Design review of the part shown in the three views and the two pictorial views. Dimensions are in mm from the part's minimum x, y and z. Coordinates: 2 decimals unless noted, no trailing zeros. Loops run counter-clockwise (first coordinate to the right, second up) from the corner with the lowest first, then second, coordinate; pieces in that order, holes last.
Q1. Wall thickness on probe 1 along X at (y, z) = (14.75, 1.5); probe 2 along Y at (x, z) = (16, 3.75); probe 3 along X at (y, z) = (12.5, 9.5): over which ranges is each line inside the solid? List them lowest first.
Q2. For P1, Ø3, axis at x = 465, y = 22.5, coming from the -Z side, flat-tipped, find the tip position at first contact; note if it passes through.
Q3. Add section C-C on x = 524. Give the boundary of the cut face in (y, z), and give its area (3 significant figures).
Q4. Add section A-A on y = 15. Give the boundary of the cut face in (x, z), and give its area (3 significant figures).
Q5. Add section B-B on z = 7.25. Give the boundary of the cut face in (x, y), and give its area (3 significant figures).
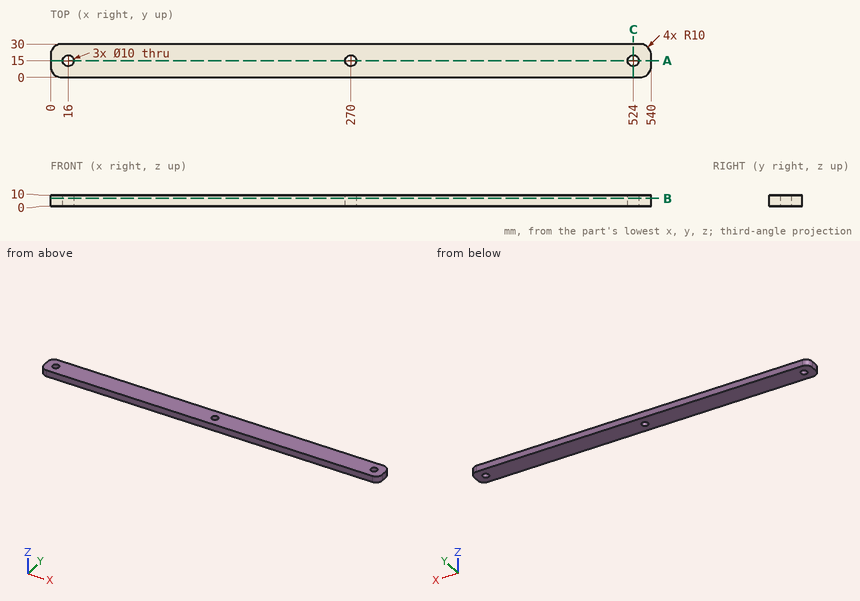
Entries:
1. probe 1: x = 0 to 11.01, 20.99 to 265.01, 274.99 to 519.01, 528.99 to 540
1. probe 2: y = 0 to 10, 20 to 30
1. probe 3: x = 0 to 11.67, 20.33 to 265.67, 274.33 to 519.67, 528.33 to 540
2. P1: stops at z = 0
3. outline: (0, 0) - (10, 0) - (10, 10) - (0, 10) - close; (20, 0) - (30, 0) - (30, 10) - (20, 10) - close
3. area: 200 mm2
4. outline: (0, 0) - (11, 0) - (11, 10) - (0, 10) - close; (21, 0) - (265, 0) - (265, 10) - (21, 10) - close; (275, 0) - (519, 0) - (519, 10) - (275, 10) - close; (529, 0) - (540, 0) - (540, 10) - (529, 10) - close
4. area: 5,100 mm2
5. outline: (0, 10) arc R10 ccw to (10, 0) - (530, 0) arc R10 ccw to (540, 10) - (540, 20) arc R10 ccw to (530, 30) - (10, 30) arc R10 ccw to (0, 20) - close; hole circle Ø10 at (16, 15); hole circle Ø10 at (270, 15); hole circle Ø10 at (524, 15)
5. area: 15,900 mm2
